Geometry: see drawing. Coordinates: mm, zero at the bounding-box minimum. A direction names the side the tool comes from. Coordinates: 2 decimals unless noted, no trailing zeros. Loops run counter-clockwise (first coordinate to the right, second up) from the corner with the lowest first, then second, coordinate; pieces in that order, holes last. Notation, with made-up numbers: (-25.75, -3.75) - (18.25, -3.75) arc R11 ccw to (18.25, 1.25) - close; hole circle Ø4 at (42.25, 66.25). An arc over 180 degrees is marked (long way). Use a Markdown table: item, result. Add a question column.
1. Section query C-C on z = 2.75. Return the cut outline in (x, y) (1 decimal).
2. Section query D-D on x = 8.75. Return the cut outline in (y, z).
3. Contact query for flat-ended pins moving along their axis: P1, Ø1.5, axis at y = 6.5, z = 3.5, coming from the -X side; P2, Ø2.5, axis at x = 12.7, y = 12.7, coming from the +Z side; P3, Ø1.5, axis at x = 16.5, z = 5, coming from the -Y side (1 decimal); P4, Ø10, axis at x = 12.7, y = 12.7, coming from the -Z side. Output: stop coordinate, or through.
4. Ray query, L1, parallel to Y at x = 12.7, z = 2.9; L2, parallel to Y at x = 12.7, z = 4.65 (1 decimal); L3, parallel to Z at x = 18.25, y = 17.5. Return the intervals inside material, ascending. Write a range as [from, to].
5. Draft query along Y for the marked faces 3, 4 and 5. Return one class per face: released by +Y, released by -Y, zero draft, split by the parting line, or undercut.
6. Access query for the marked faces 1 and 2. Directions: +Z, -Z, +X, -X, +Y, -Y. A direction counts if a zero-diameter tool reaches every point of the face in a straight line with its end or side. Return the directions, or none.
7. Section query A-A on y = 12.7. Return the cut outline in (x, z) (1 decimal).
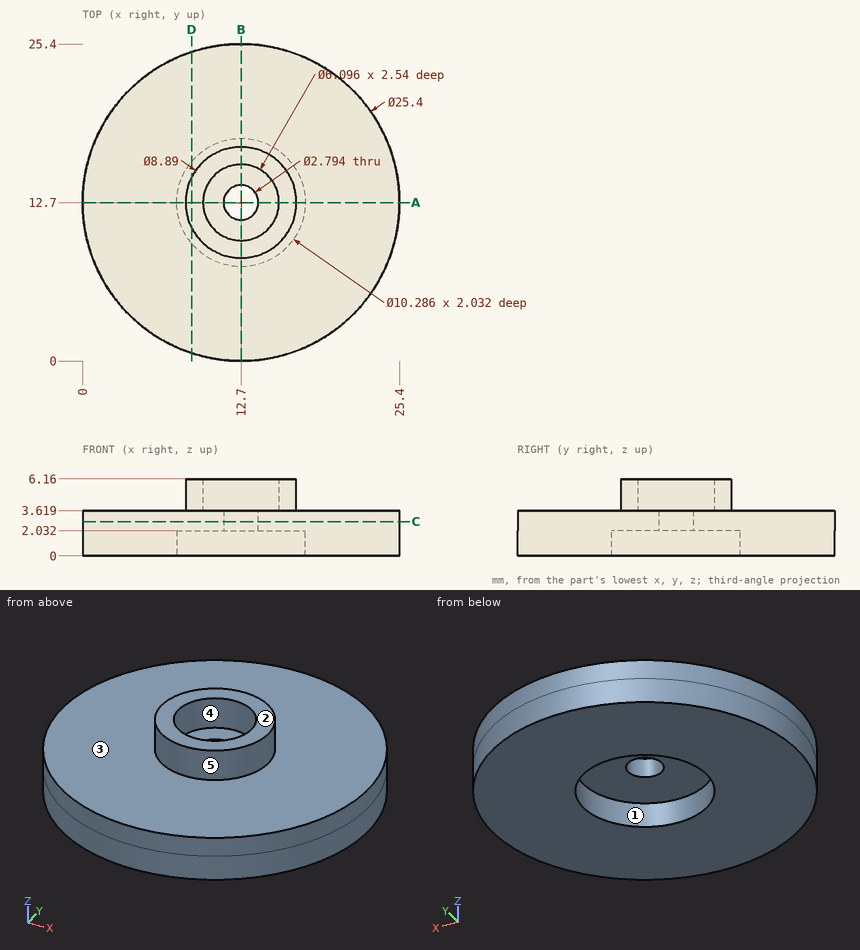
Resolved:
| question | item | result |
|---|---|---|
| 1 | outline | circle Ø25.4 at (12.7, 12.7); hole circle Ø2.8 at (12.7, 12.7) |
| 2 | outline | (0.63, 0) - (9.41, 0) - (9.41, 2.03) - (15.99, 2.03) - (15.99, 0) - (24.77, 0) - (24.77, 3.62) - (14.74, 3.62) - (14.74, 6.16) - (10.66, 6.16) - (10.66, 3.62) - (0.63, 3.62) - close |
| 3 | P1 | x = 1.23 |
| 3 | P2 | through |
| 3 | P3 | y = 9.5 |
| 3 | P4 | z = 2.03 |
| 4 | L1 | [0, 11.3], [14.1, 25.4] |
| 4 | L2 | [8.3, 9.7], [15.7, 17.1] |
| 4 | L3 | [0, 3.62] |
| 5 | face 3 | zero draft |
| 5 | face 4 | undercut |
| 5 | face 5 | split by the parting line |
| 6 | face 1 | -Z |
| 6 | face 2 | +Z, +X, -X, +Y, -Y |
| 7 | outline | (0, 0) - (7.6, 0) - (7.6, 2) - (11.3, 2) - (11.3, 3.6) - (9.7, 3.6) - (9.7, 6.2) - (8.3, 6.2) - (8.3, 3.6) - (0, 3.6) - close; (14.1, 2) - (17.8, 2) - (17.8, 0) - (25.4, 0) - (25.4, 3.6) - (17.1, 3.6) - (17.1, 6.2) - (15.7, 6.2) - (15.7, 3.6) - (14.1, 3.6) - close |
